Source: CAD feature listing. Evaluate the final solid. Frame: model axes, mm. A direction names the side the tool comes from. Give positions to 0.01 mm unless a question says otherwise; leave off trailing zeros. Order: outer loops, then holes, each group sorted by start corner. A loop starts at its lowest first (then second) coordinate and runs counter-clockwise, first axis right, second up.
Solid Edge part; units mm, degrees
sketch "Sketch1" plane through (0, 0, 0) normal (0, 0, 1) x (1, 0, 0)
  line L0 (6.8, -6.8) -> (6.8, 6.8)
  line L1 (6.8, 6.8) -> (-6.8, 6.8)
  line L2 (-6.8, 6.8) -> (-6.8, -6.8)
  line L3 (-6.8, -6.8) -> (6.8, -6.8)
  circle A0 centre (0, 0) radius 4.09
extrude "Protrusion1" add sketch "Sketch1" along normal blind 10
sketch "Sketch2" plane through (0, 0, 10) normal (0, 0, 1) x (0, 1, 0)
  circle A0 centre (0, 0) radius 4.09
  line L0 (10, -10) -> (10, 10)
  line L1 (10, 10) -> (-10, 10)
  line L2 (-10, 10) -> (-10, -10)
  line L3 (-10, -10) -> (10, -10)
extrude "ExtrudedProtrusion_2" add sketch "Sketch2" along normal blind 4
sketch "Sketch3" plane through (-6.8, 0, 5) normal (-1, 0, 0) x (0, 0, 1)
  line L0 (5, -6.7794) -> (-5, -6.7794)
  line L1 (-5, -6.7794) -> (-5, 6.7794)
  line L2 (-5, 6.7794) -> (5, 6.7794)
  line L3 (5, 6.7794) -> (5, -6.7794)
  circle A0 centre (0, 0) radius 2.75
extrude "ExtrudedProtrusion_3" add sketch "Sketch3" along normal blind 2.5
sketch "Sketch4" plane through (0, 0, 14) normal (0, 0, 1) x (0, 1, 0)
  circle A0 centre (0, 0) radius 4.09
  line L0 (10, -10) -> (10, 10)
  line L1 (10, 10) -> (-10, 10)
  line L2 (-10, 10) -> (-10, -10)
  line L3 (-10, -10) -> (10, -10)
extrude "ExtrudedProtrusion_4" add sketch "Sketch4" along normal blind 4
(1) Section C-C, the plane y = -6.25. Return loops of the section in (x, z), plus the area to 3 significant figures.
(2) Section D-D, the plane x = -5.5. Return loops of the section in (y, z), plus the area to 3 significant figures.
(3) Section B-B, the plane x = -0.5. Return loops of the section in (y, z), plus the area to 3 significant figures.
(4) Pin query (flat end, axial travel): pin 1 Ø3 at (x, z) = (-8.5, 7) entering from +Y; pin 2 Ø2 at (x, z) = (-7.5, 7) entering from -Y; pin 3 Ø3 at (y, z) = (-1.5, 2.5) entering from +X. Return the tip coordinate at first contact, or that it passes through.
(5) Line query: line 1 along X through (y, z) = (0, 13.75); line 2 along Y through (x, z) = (-7.3, 5); line 3 along X through (y, z) = (-5, 1). Output: solid intervals per line, ascending.
(6) Draft query along Z for faces 1 (the flat face through (10, 0, 14)), 2 (the flat face through (-5, 0, 0)), 3 (the flat face through (-6.8, 0, 5)), 4 (the cylindrical face through (-8.03, 1.05, 7.54)). Return one class per face: +Z half, -Z half, draft (parallel to the pull), parting line (faces both ways), or undercut.
(7) Access query for faces 5 (the flat face through (-8, 6.779, 5)), 6 (the flat face through (0, 6.8, 5)), 7 (the flat face through (0, -6.8, 5)), 8 (the flat face through (6.8, 0, 5)). Directions: +Z, -Z, +X, -X, +Y, -Y. A direction counts if a zero-diameter tool reaches every point of the face in a straight line with its end or side. Return the directions, or none.
Checks:
1. outline: (-10, 10) - (-9.3, 10) - (-9.3, 0) - (6.8, 0) - (6.8, 10) - (10, 10) - (10, 18) - (-10, 18) - close
1. area: 321 mm2
2. outline: (-10, 10) - (-6.8, 10) - (-6.8, 0) - (6.8, 0) - (6.8, 10) - (10, 10) - (10, 18) - (-10, 18) - close
2. area: 296 mm2
3. outline: (-10, 10) - (-6.8, 10) - (-6.8, 0) - (-4.06, 0) - (-4.06, 18) - (-10, 18) - close; (4.06, 0) - (6.8, 0) - (6.8, 10) - (10, 10) - (10, 18) - (4.06, 18) - close
3. area: 150 mm2
4. pin 1: stops at y = 6.78
4. pin 2: stops at y = -6.8
4. pin 3: stops at x = 6.8
5. line 1: x = -10 to -4.09, 4.09 to 10
5. line 2: y = -6.78 to -2.75, 2.75 to 6.78
5. line 3: x = -9.3 to 6.8
6. face 1: draft
6. face 2: -Z half
6. face 3: undercut
6. face 4: undercut
7. face 5: -Z, -X, +Y
7. face 6: -Z, +X, -X, +Y
7. face 7: -Z, +X, -X, -Y
7. face 8: -Z, +X, +Y, -Y
